```python
from build123d import *

# Parameters (mm, degrees)
F0_R            = 17.4625
F0_W            = 19.05
F0_H            = 6.35
F1_DEPTH        = 19.05
F2_DEPTH        = 6.35
F2_COPIES_COUNT = 4
F3_DEPTH        = 19.051
F3_COPIES_COUNT = 4


# Not quite as in the source:
# - a pattern or mirror of a feature is missing from the dataset's text; its kind, count and spacing are read off the source's solid


with BuildPart() as f1:
    # F0 (on Top) → F1 (new body)
    with BuildSketch(Plane.XY):
        with BuildLine():
            ThreePointArc((-9.525, 139.3749058296), (-95.3557746023, -102.0948884617), (139.7, 0))
            ThreePointArc((139.7, 0), (102.0948884617, 95.3557746023), (9.525, 139.3749058296))
            Line((9.525, 139.3749058296), (9.525, 120.3249058296))
            Line((9.525, 120.3249058296), (9.525, 113.9749058296))
            Line((9.525, 113.9749058296), (-9.525, 113.9749058296))
            Line((-9.525, 113.9749058296), (-9.525, 120.3249058296))
            Line((-9.525, 120.3249058296), (-9.525, 139.3749058296))
        make_face()
        with Locations((101.4398184138, 36.921074472)):
            Circle(F0_R, mode=Mode.SUBTRACT)
        with Locations((36.921074472, 101.4398184138)):
            Circle(F0_R, mode=Mode.SUBTRACT)
        with Locations((76.3321770291, 76.3321770291)):
            Circle(F0_R, mode=Mode.SUBTRACT)
        with BuildLine():
            Line((9.525, 120.3249058296), (9.525, 139.3749058296))
            ThreePointArc((9.525, 139.3749058296), (0, 139.7), (-9.525, 139.3749058296))
            Line((-9.525, 139.3749058296), (-9.525, 120.3249058296))
            Line((-9.525, 120.3249058296), (9.525, 120.3249058296))
        make_face()
        with Locations((36.921074472, 101.4398184138)):
            Circle(F0_R)
        with Locations((76.3321770291, 76.3321770291)):
            Circle(F0_R)
        with Locations((101.4398184138, 36.921074472)):
            Circle(F0_R)
        with Locations((0, 117.1499058296)):
            Rectangle(F0_W, F0_H)
    extrude(amount=-F1_DEPTH)

    # F0 (on Top) → F2 (cut)
    with BuildSketch(Plane.XY):
        with Locations((36.921074472, 101.4398184138)):
            Circle(F0_R)
        with Locations((76.3321770291, 76.3321770291)):
            Circle(F0_R)
        with Locations((101.4398184138, 36.921074472)):
            Circle(F0_R)
    f2 = extrude(amount=-F2_DEPTH, mode=Mode.SUBTRACT)

    # F2_copies: F2 ×4 about axis
    f2_copies_axis = Axis((0, 0, 0), (0, 0, 1))
    for i in range(1, F2_COPIES_COUNT):
        add(f2.rotate(f2_copies_axis, i * 360 / F2_COPIES_COUNT), mode=Mode.SUBTRACT)

    # F0 (on Top) → F3 (cut, through all)
    with BuildSketch(Plane.XY):
        with BuildLine():
            Line((9.525, 120.3249058296), (9.525, 139.3749058296))
            ThreePointArc((9.525, 139.3749058296), (0, 139.7), (-9.525, 139.3749058296))
            Line((-9.525, 139.3749058296), (-9.525, 120.3249058296))
            Line((-9.525, 120.3249058296), (9.525, 120.3249058296))
        make_face()
    f3 = extrude(amount=-F3_DEPTH, mode=Mode.SUBTRACT)

    # F3_copies: F3 ×4 about axis
    f3_copies_axis = Axis((0, 0, 0), (0, 0, 1))
    for i in range(1, F3_COPIES_COUNT):
        add(f3.rotate(f3_copies_axis, i * 360 / F3_COPIES_COUNT), mode=Mode.SUBTRACT)


solid = f1.part
```
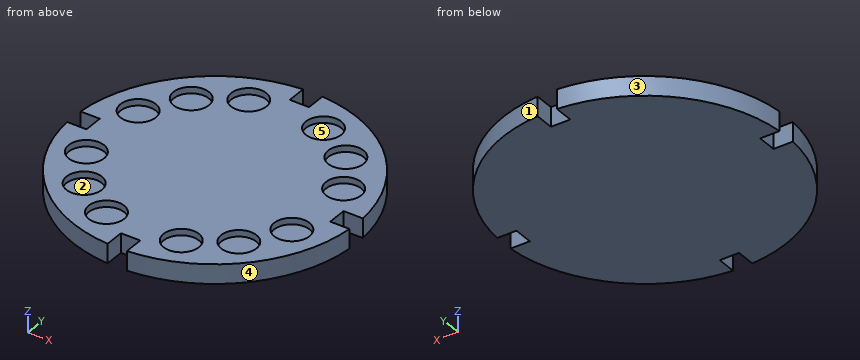
The model under review builds one solid part; all positions refer to its coordinate system, in mm. Face numbers are marked on the shaded views. A direction names the side the tool comes from. Round coordinates to 2 decimals unless told otherwise and drop trailing zeros. Write each loop counter-clockwise with the first axis right and the second up, starting at its lowest first coordinate (ties: lowest second). Pieces come first, ordered by that corner, then holes.
(1) Insertion check: pin 1 (8 mm diameter, centred on x = -88.5, z = -11.5, fed in from -Y); pin 2 (3 mm diameter, centred on x = 38.5, z = -13, fed in from +Y); pin 3 (10.5 mm diameter, centred on x = 45, y = 103.5, fed in from +Z). Each pin has a flat end and moves straight along its axis. Give the tip position at first contact, or say it passes through.
(2) We need section C-C on x = 66.5. Give the boundary of the cut face in (y, z), and give its area (3 significant figures).
(3) Wall thickness on L1, parallel to X at y = 106, z = -2.25 (3 decimals); L2, parallel to X at y = 48.5, z = -4.5; L3, parallel to Y at x = -111, z = -6.25: over which ranges is each line inside the solid? List them lowest first.
(4) Mouldability with a two-part tool opening along Y and no side actions: class the marked faces 3, 4 and 5 as +Y half, -Y half, draft (parallel to the pull), parting line (faces both ways), or undercut.
(5) We need section A-A on z = -10.25. Give the boundary of the cut face in (x, y) (3 decimals).
(6) Machinability: for the marked faces 1 and 2, which of the approach directions +Z, -Z, +X, -X, +Y, -Y give a long, thin tool a straight path to every point of the face, cutting with its end or side? Answer none if there is none.
(7) We need section B-B on y = -105. Give the boundary of the cut face in (x, z), and give its area (3 significant figures).
Findings below:
1. pin 1: stops at y = -111.25
1. pin 2: stops at y = 134.71
1. pin 3: stops at z = -6.35
2. outline: (-122.86, -19.05) - (122.86, -19.05) - (122.86, 0) - (90.76, 0) - (90.76, -6.35) - (61.9, -6.35) - (61.9, 0) - (-61.9, 0) - (-61.9, -6.35) - (-90.76, -6.35) - (-90.76, 0) - (-122.86, 0) - close
2. area: 4,310 mm2
3. L1: x = -90.995 to -53.778, -20.065 to 20.065, 53.778 to 90.995
3. L2: x = -131.01 to -114.51, -88.37 to 88.37, 114.51 to 131.01
3. L3: y = -84.82 to -51.53, -22.31 to 22.31, 51.53 to 84.82
4. face 3: +Y half
4. face 4: -Y half
4. face 5: undercut
5. outline: (-139.375, -9.525) arc R139.7 ccw to (-9.525, -139.375) - (-9.525, -120.325) - (9.525, -120.325) - (9.525, -139.375) arc R139.7 ccw to (139.375, -9.525) - (120.325, -9.525) - (120.325, 9.525) - (139.375, 9.525) arc R139.7 ccw to (9.525, 139.375) - (9.525, 120.325) - (-9.525, 120.325) - (-9.525, 139.375) arc R139.7 ccw to (-139.375, 9.525) - (-120.325, 9.525) - (-120.325, -9.525) - close
6. face 1: +Z, -Z, +X, +Y
6. face 2: +Z
7. outline: (-92.15, -19.05) - (92.15, -19.05) - (92.15, 0) - (54.02, 0) - (54.02, -6.35) - (19.83, -6.35) - (19.83, 0) - (-19.83, 0) - (-19.83, -6.35) - (-54.02, -6.35) - (-54.02, 0) - (-92.15, 0) - close
7. area: 3,080 mm2
